```python
from build123d import *

# Parameters (mm, degrees)
SKETCH1_R           = 2.5
BOSS_EXTRUDE1_DEPTH = 3
FILLET1_R           = 5
FILLET2_R           = 5
FILLET4_R           = 9.2


with BuildPart() as part:
    # Sketch1 → Boss-Extrude1 (new body)
    with BuildSketch(Plane.XY):
        Polygon((53, 53), (53, 18.4), (83, 18.4), (83, 0), (0, 0), (0, 53), align=None)
        with Locations((76.6, 9.2)):
            Circle(SKETCH1_R, mode=Mode.SUBTRACT)
    extrude(amount=BOSS_EXTRUDE1_DEPTH)

    # Fillet1
    fillet1_edges = [part.edges().sort_by_distance(p)[0] for p in [
        (0, 53, 1.5),
        (53, 53, 1.5),
        (0, 0, 1.5),
    ]]
    fillet(fillet1_edges, radius=FILLET1_R)

    # Fillet2
    fillet2_edges = [part.edges().sort_by_distance(p)[0] for p in [
        (53, 18.4, 1.5),
    ]]
    fillet(fillet2_edges, radius=FILLET2_R)

    # Fillet4
    fillet4_edges = [part.edges().sort_by_distance(p)[0] for p in [
        (83, 0, 1.5),
        (83, 18.4, 1.5),
    ]]
    fillet(fillet4_edges, radius=FILLET4_R - 0.0001)  # a hair under: the kernel refuses the full size


solid = part.part
```
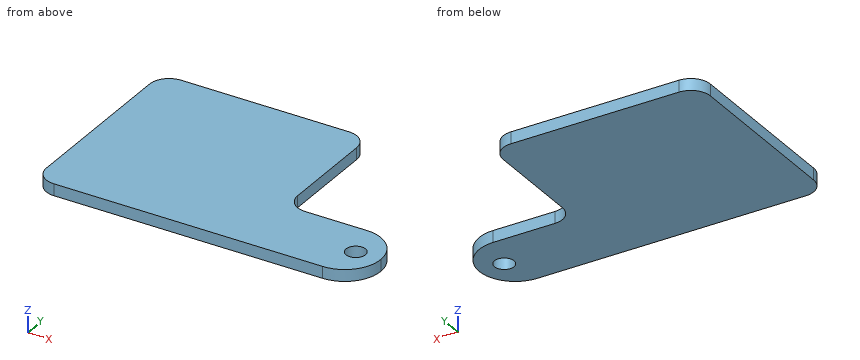
Geometry: final body of the model. Coordinates: model frame, mm. Coordinates: 2 decimals unless noted, no trailing zeros. Loops run counter-clockwise (first coordinate to the right, second up) from the corner with the lowest first, then second, coordinate; pieces in that order, holes last. Notation, with made-up numbers: M -9.5,64.25 L 0.5,64.25 A15 ccw 0.5,89.25 Z; hole C 80,15.25 d9. An arc over 180 degrees is marked long. Put each result on its own line as item: value.
(1) Cut plane D-D on x = 64. Return the cut outline in (y, z), then the cut area to 3 significant figures.
Answer sheet:
outline: M 0,0 L 18.4,0 L 18.4,3 L 0,3 Z
area: 55.2 mm^2
(2) First-contact query: pin 1 (10 mm diameter, centred on x = 52, y = 34, fed in from -Z). Flat tip, straight axial feed; report the tip coordinate or a pass-through.
Answer sheet:
pin 1: stops at z = 0
(3) Cut plane C-C on y = 40. Return the cut outline in (x, z), then the cut area to 3 significant figures.
Answer sheet:
outline: M 0,0 L 53,0 L 53,3 L 0,3 Z
area: 159 mm^2
(4) Material intervals for probe 1 along X at (y, z) = (25, 0.85); probe 2 along Y at (x, z) = (76.6, 1.8); probe 3 along Y at (x, z) = (61.5, 1.05), sorted ascending.
Answer sheet:
probe 1: x = 0 to 53
probe 2: y = 0.44 to 6.7, 11.7 to 17.96
probe 3: y = 0 to 18.4
(5) Cut plane B-B on x = 76.6. Return the cut outline in (y, z).
Answer sheet:
outline: M 0.44,0 L 6.7,0 L 6.7,3 L 0.44,3 Z; M 11.7,0 L 17.96,0 L 17.96,3 L 11.7,3 Z
